The listing builds one solid part. Answer for the finished solid, in the listing's coordinates (mm). Round coordinates to 2 decimals unless told otherwise and drop trailing zeros.
(1) Find the intervals of material crossed by probe 1 along X at (y, z) = (6.5, 0); probe 2 along Y at (x, z) = (0.1, -0.1), in increasing order.
(2) This flat-tipped pin is pushed along its axis until it touches: pin 1 Ø1 at (x, y) = (-0.5, 1) entering from -Z. Where does it stop, or does it pass through?
(3) The mould has two halves that part along X. Classify faces 1 (the face through (-0.225, 4.849, 0.715)), 2 (the face through (0, 8.83, 0)): +X half, -X half, draft (parallel to the pull), parting line (faces both ways), or undercut.
from build123d import *

# Parameters (mm, degrees)
CUT_EXTRUDE1_DEPTH = 0.2


with BuildPart() as part:
    # Sketch1 → Revolve1 (revolve)
    with BuildSketch(Plane.XY, mode=Mode.PRIVATE) as revolve1_sk:
        Polygon((0, 0), (0.75, 0.755428016), (0.75, 8.83), (1.03, 9.03), (0, 9.03), align=None)
    revolve(revolve1_sk.sketch.rotate(Axis((0, 12.912548638, 0), (0, -1, 0)), 90), axis=Axis((0, 12.912548638, 0), (0, -1, 0)))

    # Sketch2 → Cut-Extrude1 (cut)
    with BuildSketch(Plane(origin=(0, 9.03, 0), x_dir=(1, 0, 0), z_dir=(0, 1, 0))):
        Polygon((-0.14, 0.14), (-0.14, 0.7), (0.14, 0.7), (0.14, 0.14), (0.7, 0.14), (0.7, -0.14), (0.14, -0.14), (0.14, -0.7), (-0.14, -0.7), (-0.14, -0.14), (-0.7, -0.14), (-0.7, 0.14), align=None)
    extrude(amount=-CUT_EXTRUDE1_DEPTH, mode=Mode.SUBTRACT)


solid = part.part
Solutions:
1. probe 1: x = -0.75 to 0.75
1. probe 2: y = 0.14 to 8.83
2. pin 1: stops at z = -0.75
3. face 1: parting line
3. face 2: undercut
